from build123d import *

# Parameters (mm, degrees)
BOX039_W        = 68
BOX039_H        = 54
BOX039_DEPTH    = 4.1
BOX038_W        = 74
BOX038_H        = 60
BOX038_DEPTH    = 4.1
CHAMFER021_SIZE = 2
CHAMFER022_SIZE = 2
BOX033_W        = 72
BOX033_H        = 58
BOX033_DEPTH    = 42
BOX032_W        = 74
BOX032_H        = 60
BOX032_DEPTH    = 42
CHAMFER020_SIZE = 0.99


with BuildPart() as obj1:
    # Box039 → Box039 (new body)
    with BuildSketch(Plane(origin=(3, -57, 0), x_dir=(1, 0, 0), z_dir=(0, 0, 1))):
        with Locations((34, 27)):
            Rectangle(BOX039_W, BOX039_H)
    extrude(amount=BOX039_DEPTH)


with BuildPart() as chamfer022:
    # Box038 → Box038 (new body)
    with BuildSketch(Plane(origin=(0, -60, 0), x_dir=(1, 0, 0), z_dir=(0, 0, 1))):
        with Locations((37, 30)):
            Rectangle(BOX038_W, BOX038_H)
    extrude(amount=BOX038_DEPTH)

    # Cut019: cut obj1
    add(obj1.part, mode=Mode.SUBTRACT)


with BuildPart() as chamfer022_1:
    # Cut019 placement: moved
    add(chamfer022.part.moved(Location((0, 0, 36.9))))

    # Chamfer021
    chamfer021_edges = [chamfer022_1.edges().sort_by_distance(p)[0] for p in [
        (37, -3, 41),
        (3, -30, 41),
        (37, -57, 41),
        (71, -30, 41),
    ]]
    chamfer(chamfer021_edges, length=CHAMFER021_SIZE)

    # Chamfer022
    chamfer022_edges = [chamfer022_1.edges().sort_by_distance(p)[0] for p in [
        (37, -3, 36.9),
        (3, -30, 36.9),
        (71, -30, 36.9),
        (37, -57, 36.9),
    ]]
    chamfer(chamfer022_edges, length=CHAMFER022_SIZE)


with BuildPart() as obj2:
    # Box033 → Box033 (new body)
    with BuildSketch(Plane(origin=(1, -59, 0), x_dir=(1, 0, 0), z_dir=(0, 0, 1))):
        with Locations((36, 29)):
            Rectangle(BOX033_W, BOX033_H)
    extrude(amount=BOX033_DEPTH)


with BuildPart() as form:
    # Box032 → Box032 (new body)
    with BuildSketch(Plane(origin=(0, -60, 0), x_dir=(1, 0, 0), z_dir=(0, 0, 1))):
        with Locations((37, 30)):
            Rectangle(BOX032_W, BOX032_H)
    extrude(amount=BOX032_DEPTH)

    # Cut014: cut obj2
    add(obj2.part, mode=Mode.SUBTRACT)

    # Chamfer020
    chamfer020_edges = [form.edges().sort_by_distance(p)[0] for p in [
        (37, -1, 42),
        (1, -30, 42),
        (37, -59, 42),
        (73, -30, 42),
    ]]
    chamfer(chamfer020_edges, length=CHAMFER020_SIZE)

    # Fusion: union Chamfer022
    add(chamfer022_1.part)


solid = form.part
Source: CAD feature listing. Evaluate the final solid. Frame: model axes, mm. A direction names the side the tool comes from. Round coordinates to 2 decimals unless told otherwise and drop trailing zeros. Loops run counter-clockwise (first coordinate to the right, second up) from the corner with the lowest first, then second, coordinate; pieces in that order, holes last. Notation, with made-up numbers: M 5,33 L 23,33 A28 cw 23,53 Z; hole C -18.5,41.5 d4. An arc over 180 degrees is marked long. Answer as CSV lines item,"result".
Q1. Line query: line 1 along Y through (x, z) = (6.5, 13); line 2 along X through (y, z) = (-57, 26.5); line 3 along Y through (x, z) = (6.5, 37.5). Output: solid intervals per line, ascending.
Verdict:
line 1,"y = -60 to -59, -1 to 0"
line 2,"x = 0 to 1, 73 to 74"
line 3,"y = -60 to -58.4, -1.6 to 0"
Q2. Reachability of faces 1 (the face through (36, -2, 40)), 2 (the face through (73, -30, 18)), 3 (the face through (36, -60, 21)) from +Z, -Z, +X, -X, +Y, -Y: full face, straight path, thin tool, end or side. Return the list, or none.
Verdict:
face 1,"+Z"
face 2,"-Z"
face 3,"+Z, -Z, +X, -X, -Y"
Q3. Cut plane B-B (z = 17.5). Return the cut outline in (x, y).
Verdict:
outline,"M 0,-60 L 74,-60 L 74,0 L 0,0 Z; hole M 1,-59 L 73,-59 L 73,-1 L 1,-1 Z"
Q4. Contact query for a flat-ended pin moving along its axis: pin 1 (12 mm diameter, centred on x = 63, y = -46, fed in from -Z). Output: stop coordinate, or through.
Verdict:
pin 1,"passes through"
Q5. Pull-direction query (X, two-part tool) for faces 4 (the face through (0, -30, 21)), 5 (the face through (36, -59, 18)), 6 (the face through (74, -30, 21)); classes: +X half, -X half, draft (parallel to the pull), parting line (faces both ways), or undercut.
Verdict:
face 4,"-X half"
face 5,"undercut"
face 6,"+X half"
